Geometry check sheet. Reference: the model listing, model coordinates, mm. Face numbers are marked on the shaded views. A direction names the side the tool comes from. Coordinates: 2 decimals unless noted, no trailing zeros. Loops run counter-clockwise (first coordinate to the right, second up) from the corner with the lowest first, then second, coordinate; pieces in that order, holes last. Notation, with made-up numbers: M 12,-5.75 L 59,-5.75 A36 cw 59,33.25 Z; hole C 56,47 d3. An arc over 180 degrees is marked long. Use CSV: the item, a comma, the result in double quotes.
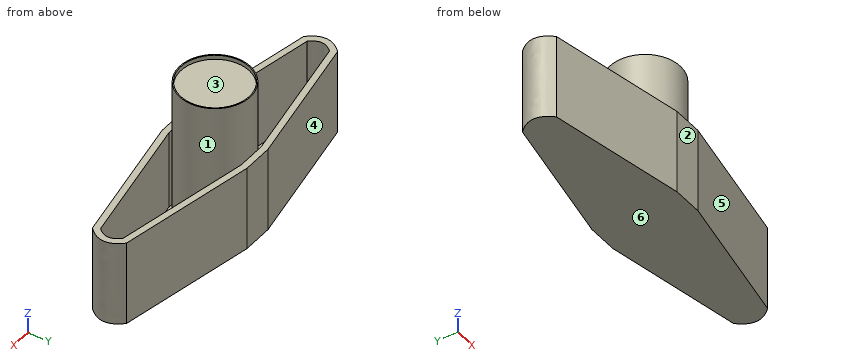
```python
from build123d import *

# Parameters (mm, degrees)
BOSS_EXTRUDE1_DEPTH = 20
SHELL2_T            = -1.5
SKETCH4_R           = 8.25
BOSS_EXTRUDE6_DEPTH = 33
SKETCH5_R           = 8
CUT_EXTRUDE1_DEPTH  = 1


with BuildPart() as part:
    # Sketch1 → Boss-Extrude1 (new body)
    with BuildSketch(Plane.XY):
        with BuildLine():
            Line((-35.5, 4), (-3.5, 10))
            Line((-3.5, 10), (3.5, 10))
            Line((3.5, 10), (35.5, 4))
            add(Edge.make_bspline(
                [(35.5, 4), (39.5, 0), (35.5, -4)],
                knots=[0, 0, 0, 1, 1, 1], degree=2))
            Line((35.5, -4), (3.5, -10))
            Line((3.5, -10), (-3.5, -10))
            Line((-3.5, -10), (-35.5, -4))
            add(Edge.make_bspline(
                [(-35.5, 4), (-39.5, 0), (-35.5, -4)],
                knots=[0, 0, 0, 1, 1, 1], degree=2))
        make_face()
    extrude(amount=BOSS_EXTRUDE1_DEPTH)

    # Shell2
    shell2_openings = [part.faces().sort_by_distance(p)[0] for p in [
        (0, 0, 20),
    ]]
    offset(amount=SHELL2_T, openings=shell2_openings, kind=Kind.INTERSECTION)

    # Sketch4 → Boss-Extrude6 (add)
    with BuildSketch(Plane.XY.offset(1.5)):
        Circle(SKETCH4_R)
    extrude(amount=BOSS_EXTRUDE6_DEPTH)

    # Sketch5 → Cut-Extrude1 (cut)
    with BuildSketch(Plane.XY.offset(34.5)):
        Circle(SKETCH5_R)
    extrude(amount=-CUT_EXTRUDE1_DEPTH, mode=Mode.SUBTRACT)


solid = part.part
```
1. Gauge pin test, flat ends, axial feed: P1, Ø10, axis at x = 4, z = 4, coming from the +Y side; P2, Ø1.5, axis at x = 8, y = -6, coming from the +Z side; P3, Ø5, axis at x = -17, z = 15.5, coming from the -Y side; P4, Ø1, axis at y = -1.5, z = 4, coming from the +X side (3 decimals). Record the tip position at first contact, or that the pin passes through.
The answers:
P1,"y = 10"
P2,"z = 1.5"
P3,"y = -7.94"
P4,"x = 37.375"
2. Section check B-B, the plane x = 0. Record the cut outline in (y, z), plus the area to 3 significant figures.
The answers:
outline,"M -10,0 L 10,0 L 10,20 L 8.5,20 L 8.5,1.5 L 8.25,1.5 L 8.25,34.5 L 8,34.5 L 8,33.5 L -8,33.5 L -8,34.5 L -8.25,34.5 L -8.25,1.5 L -8.5,1.5 L -8.5,20 L -10,20 Z"
area,"614 mm^2"
3. Set-up check for the marked faces 1 and 2: record each of +Z, -Z, +X, -X, +Y, -Y from which the full face is reachable in a straight line by a thin tool's end or side.
The answers:
face 1,"+Z"
face 2,"+Z, -Z, +X, -X, -Y"
4. Release check for a two-part mould opening along Y. For the marked faces 3, 4, 5 and 6 record: +Y half, -Y half, draft (parallel to the pull), parting line (faces both ways), or undercut.
The answers:
face 3,"undercut"
face 4,"+Y half"
face 5,"-Y half"
face 6,"draft"
5. Section check C-C, the plane y = 6. Record the cut outline in (x, z).
The answers:
outline,"M -24.83,0 L 24.83,0 L 24.83,20 L 16.69,20 L 16.69,1.5 L 5.66,1.5 L 5.66,34.5 L 5.29,34.5 L 5.29,33.5 L -5.29,33.5 L -5.29,34.5 L -5.66,34.5 L -5.66,1.5 L -16.69,1.5 L -16.69,20 L -24.83,20 Z"
6. Thickness scan on line 1 (Y direction, x = 0, z = 34.2); line 2 (X direction, y = 1.25, z = 7.5); line 3 (Z direction, x = -20.5, y = 3.5). Record the ranges inside material, lowest first. Write a range as [from, to].
The answers:
line 1,"[-8.25, -8], [8, 8.25]"
line 2,"[-37.3, -35.7], [-8.15, 8.15], [35.7, 37.3]"
line 3,"[0, 1.5]"
7. Section check D-D, the plane z = 31. Record the cut outline in (x, y).
The answers:
outline,"C 0,0 d16.5"
8. Section check A-A, the plane z = 4. Count the separate pieces of the cut face and the enclosed holes in it, plus the area to 3 significant figures.
The answers:
separate pieces,"2"
enclosed holes,"1"
area,"451 mm^2"
